```python
from build123d import *

# Parameters (mm, degrees)
F0_W      = 279.4
F0_H      = 203.2
F1_DEPTH  = 203.2
F5_W      = 228.6
F5_H      = 152.4
F6_DEPTH  = 152.4
F2_R      = 3.175
F2_R_2    = 1.8288
F7_DEPTH  = 25.4
F3_R      = 6.35
F8_DEPTH  = 25.4
F4_R      = 6.35
F9_DEPTH  = 25.4
F10_R     = 6.35
F11_DEPTH = 254


with BuildPart() as f1:
    # F0 (on Front) → F1 (new body)
    with BuildSketch(Plane.XZ):
        Rectangle(F0_W, F0_H)
    extrude(amount=-F1_DEPTH)

    # F5 (on Front) → F6 (cut)
    with BuildSketch(Plane.XZ):
        Rectangle(F5_W, F5_H)
    extrude(amount=-F6_DEPTH, mode=Mode.SUBTRACT)

    # F2 (on face) → F7 (cut)
    with BuildSketch(Plane.XY.offset(101.6)):
        with Locations((0, 101.6)):
            Circle(F2_R)
        with Locations((28.575, 101.6)):
            Circle(F2_R_2)
    extrude(amount=-F7_DEPTH, mode=Mode.SUBTRACT)

    # F3 (on face) → F8 (cut)
    with BuildSketch(Plane.YZ.offset(139.7)):
        with Locations((101.6, 0)):
            Circle(F3_R)
    extrude(amount=-F8_DEPTH, mode=Mode.SUBTRACT)

    # F4 (on face) → F9 (cut)
    with BuildSketch(Plane(origin=(-139.7, 0, 0), x_dir=(0, -1, 0), z_dir=(-1, 0, 0))):
        with Locations((-101.6, 0)):
            Circle(F4_R)
    extrude(amount=-F9_DEPTH, mode=Mode.SUBTRACT)

    # F10 (on Front) → F11 (cut)
    with BuildSketch(Plane.XZ):
        with Locations((62.176916, 0)):
            Circle(F10_R)
    extrude(amount=-F11_DEPTH, mode=Mode.SUBTRACT)


solid = f1.part
```
Could you check a few things on this model? Use its own coordinates, in mm. A direction names the side the tool comes from. Give positions to 0.01 mm unless a question says otherwise; leave off trailing zeros. Write each loop counter-clockwise with the first axis right and the second up, starting at its lowest first coordinate (ties: lowest second). Pieces come first, ordered by that corner, then holes. Notation, with made-up numbers: (-32.75, 28) - (12.25, 28) arc R6 cw to (12.25, 36) - close; hole circle Ø1 at (-1.75, 66.25). An arc over 180 degrees is marked (long way). One line per item, written item: value. Start each with the question number.
Item 1: Imagine slicing it at B-B, the plane z = 0. List the corners of the cut face in (x, y) for me, and give its area (3 significant figures).
Item 2: If we mould it in two halves opening along Z, with no side actions, what happens to faces 4 (the face through (-2, 100, -101.6)), 5 (the face through (-2, 203.2, 1)), 6 (the face through (-114.3, 75, -1))? For each: +Z half, -Z half, draft (parallel to the pull), parting line (faces both ways), or undercut.
Item 3: Imagine slicing it at C-C, the plane y = 136.5. List the corners of the cut face in (x, z) for me, and give its area (3 significant figures).
Item 4: I'm going to push flat-ended pins straight in: pin 1 (10 mm diameter, centred on x = 62.18, z = 0, fed in from +Y); pin 2 (2 mm diameter, centred on x = 72, z = 72.5, fed in from -Y). Where does each tip first touch, or does it pass through?
Item 5: Imagine slicing it at A-A, the plane x = 110.5. List the corners of the cut face in (y, z) for me, and give its area (3 significant figures).
Item 6: Please list where these lines run through material, in increasing order: line 1 (Z direction, x = -26.5, y = 30.5); line 2 (X direction, y = 116.5, z = -31); line 3 (Z direction, x = 128, y = 101). Write a range as from..to.
Item 7: Which directions (+Z, -Z, +X, -X, +Y, -Y) give clear straight access to the entire face, cutting with the end or side of a thin tool? Please do faces 1 (the face through (-2, 75, -76.2)), 2 (the face through (1.707, 104.277, 89.078)), 3 (the face through (139.7, 123, -1)).
Item 8: Imagine slicing it at D-D, the plane z = 30. List the corners of the cut face in (x, y) for me.
Geometry says:
1. outline: (-139.7, 0) - (-114.3, 0) - (-114.3, 95.25) - (-139.7, 95.25) - close; (-139.7, 107.95) - (-114.3, 107.95) - (-114.3, 152.4) - (55.83, 152.4) - (55.83, 203.2) - (-139.7, 203.2) - close; (68.53, 152.4) - (114.3, 152.4) - (114.3, 107.95) - (139.7, 107.95) - (139.7, 203.2) - (68.53, 203.2) - close; (114.3, 0) - (139.7, 0) - (139.7, 95.25) - (114.3, 95.25) - close
1. area: 20,600 mm^2
2. face 4: -Z half
2. face 5: draft
2. face 6: undercut
3. outline: (-139.7, -101.6) - (139.7, -101.6) - (139.7, 101.6) - (-139.7, 101.6) - close; hole (-114.3, -76.2) - (114.3, -76.2) - (114.3, 76.2) - (-114.3, 76.2) - close
3. area: 21,900 mm^2
4. pin 1: through
4. pin 2: y = 152.4
5. outline: (0, -101.6) - (203.2, -101.6) - (203.2, 101.6) - (0, 101.6) - (0, 76.2) - (152.4, 76.2) - (152.4, -76.2) - (0, -76.2) - close
5. area: 18,100 mm^2
6. line 1: -101.6..-76.2, 76.2..101.6
6. line 2: -139.7..-114.3, 114.3..139.7
6. line 3: -101.6..-6.32, 6.32..101.6
7. face 1: -Y
7. face 2: +Z
7. face 3: +Z, -Z, +X, +Y, -Y
8. outline: (-139.7, 0) - (-114.3, 0) - (-114.3, 152.4) - (114.3, 152.4) - (114.3, 0) - (139.7, 0) - (139.7, 203.2) - (-139.7, 203.2) - close
